from build123d import *

# Parameters (mm, degrees)
SKETCH1_R           = 12.5
SKETCH1_W           = 100
SKETCH1_H           = 75
BOSS_EXTRUDE1_DEPTH = 20


with BuildPart() as part:
    # Sketch1 → Boss-Extrude1 (new body)
    with BuildSketch(Plane.XY):
        with BuildLine():
            Line((-75, 60), (75, 60))
            ThreePointArc((75, 60), (135, 0), (75, -60))
            Line((75, -60), (-75, -60))
            ThreePointArc((-75, -60), (-135, 0), (-75, 60))
        make_face()
        with Locations((75, 0)):
            Circle(SKETCH1_R, mode=Mode.SUBTRACT)
        with Locations((-75, 0)):
            Circle(SKETCH1_R, mode=Mode.SUBTRACT)
        Rectangle(SKETCH1_W, SKETCH1_H, mode=Mode.SUBTRACT)
    extrude(amount=BOSS_EXTRUDE1_DEPTH)


solid = part.part
Geometry: final body of the model. Coordinates: model frame, mm. A direction names the side the tool comes from. Coordinates: 2 decimals unless noted, no trailing zeros. Loops run counter-clockwise (first coordinate to the right, second up) from the corner with the lowest first, then second, coordinate; pieces in that order, holes last. Notation, with made-up numbers: (-7, 15) - (44, 15) arc R23 ccw to (44, 35) - close; hole circle Ø8 at (87, -11). An arc over 180 degrees is marked (long way). Put each result on its own line as item: value. Start each with the question number.
Q1. Cut plane A-A, the plane y = 0. Return loops of the section in (x, z), and give its area (3 significant figures).
Q2. Set-up query: faces 4 (the flat face through (50, -1, 10)), 5 (the cylindrical face through (134.985, 1.319, 9.86)). Return all of +Z, -Z, +X, -X, +Y, -Y with unobstructed straight access to the full face (end or side cutting, diameter ignored); none if empty.
Q3. Pin query (flat end, axial travel): pin 1 Ø1 at (x, z) = (92.5, 12.5) entering from -Y; pin 2 Ø15 at (x, y) = (75, 0) entering from -Z; pin 3 Ø10 at (y, z) = (37.5, 7.5) entering from +X; pin 4 Ø6 at (y, z) = (-4.5, 5.5) entering from -X. Return the tip coordinate at first contact, or that it passes through.
Q4. Cut plane C-C, the plane z = 9. Return loops of the section in (x, y), and give its area (3 significant figures).
Q5. Cut plane D-D, the plane y = 24. Return loops of the section in (x, z), and give its area (3 significant figures).
Q6. Pull-direction query (X, two-part tool) for faces 1 (the cylindrical face through (62.512, 0.55, 9.86)), 2 (the flat face through (-1, 60, 10)), 3 (the cylindrical face through (-134.985, -1.319, 9.86)); classes: released by +X, released by -X, zero draft, split by the parting line, or undercut.
Q7. Cut plane B-B, the plane x = 10. Return loops of the section in (y, z), and give its area (3 significant figures).
Q8. Line query: line 1 (Y direction, x = 75, z = 14.25); line 2 (Y direction, x = -26, z = 7.75); line 3 (X direction, y = -26, z = 3.25). Output: solid intervals per line, ascending.
Filled sheet:
1. outline: (-135, 0) - (-87.5, 0) - (-87.5, 20) - (-135, 20) - close; (-62.5, 0) - (-50, 0) - (-50, 20) - (-62.5, 20) - close; (50, 0) - (62.5, 0) - (62.5, 20) - (50, 20) - close; (87.5, 0) - (135, 0) - (135, 20) - (87.5, 20) - close
1. area: 2,400 mm²
2. face 4: +Z, -Z
2. face 5: +Z, -Z, +X
3. pin 1: y = -57.54
3. pin 2: through
3. pin 3: x = 125.44
3. pin 4: x = -134.98
4. outline: (-75, -60) - (75, -60) arc R60 ccw to (75, 60) - (-75, 60) arc R60 ccw to start; hole circle Ø25 at (-75, 0); hole (-50, -37.5) - (50, -37.5) - (50, 37.5) - (-50, 37.5) - close; hole circle Ø25 at (75, 0)
4. area: 20,800 mm²
5. outline: (-129.99, 0) - (-50, 0) - (-50, 20) - (-129.99, 20) - close; (50, 0) - (129.99, 0) - (129.99, 20) - (50, 20) - close
5. area: 3,200 mm²
6. face 1: undercut
6. face 2: zero draft
6. face 3: released by -X
7. outline: (-60, 0) - (-37.5, 0) - (-37.5, 20) - (-60, 20) - close; (37.5, 0) - (60, 0) - (60, 20) - (37.5, 20) - close
7. area: 900 mm²
8. line 1: -60 to -12.5, 12.5 to 60
8. line 2: -60 to -37.5, 37.5 to 60
8. line 3: -129.07 to -50, 50 to 129.07
